The model under review builds one solid part; all positions refer to its coordinate system, in mm. Round coordinates to 2 decimals unless told otherwise and drop trailing zeros. Loops run counter-clockwise (first coordinate to the right, second up) from the corner with the lowest first, then second, coordinate; pieces in that order, holes last. Notation, with made-up numbers: (23.25, 60) - (43.25, 60) arc R25 ccw to (43.25, 95) - close; hole circle Ø6 at (-37.5, 61). An arc over 180 degrees is marked (long way). Answer as CSV lines item,"result".
from build123d import *

# Parameters (mm, degrees)
F0_R     = 76.194135209
F1_DEPTH = 15.24
F2_DEPTH = 15.24
F3_R     = 5.08
F5_DEPTH = 0.762
F6_R     = 71.114135209
F7_DEPTH = 0.254


with BuildPart() as f1:
    # F0 (on Front) → F1 (new body)
    with BuildSketch(Plane.XZ):
        Circle(F0_R)
    extrude(amount=F1_DEPTH)

    # F2 (add): a face of the model
    f2_faces = [f1.faces().sort_by_distance(p)[0] for p in [
        (0, 0, 0),
    ]]
    extrude(f2_faces, amount=F2_DEPTH)

    # F3
    f3_edges = [f1.edges().sort_by_distance(p)[0] for p in [
        (76.194135, -7.62, 0),
        (-76.194135, 0, 0),
        (-76.194135, -15.24, 0),
        (76.194135, 7.62, 0),
        (-76.194135, 15.24, 0),
    ]]
    fillet(f3_edges, radius=F3_R)

    # F4 (on face) → F5 (join)
    with BuildSketch(Plane.XZ.offset(15.24)):
        with BuildLine():
            Line((61.5866476591, -35.5570676045), (0, 0))
            Line((0, 0), (-61.5866476591, -35.5570676045))
            ThreePointArc((-61.5866476591, -35.5570676045), (0, -71.114135209), (61.5866476591, -35.5570676045))
        make_face()
        with BuildLine():
            Line((-61.5866476591, -35.5570676045), (0, 0))
            Line((0, 0), (0, 71.114135209))
            ThreePointArc((0, 71.114135209), (-61.5866476591, 35.5570676045), (-61.5866476591, -35.5570676045))
        make_face()
        with BuildLine():
            Line((0, 71.114135209), (0, 0))
            Line((0, 0), (61.5866476591, -35.5570676045))
            ThreePointArc((61.5866476591, -35.5570676045), (68.6909798125, -18.4056925681), (71.114135209, 0))
            ThreePointArc((71.114135209, 0), (50.2852872445, 50.2852872445), (0, 71.114135209))
        make_face()
    extrude(amount=F5_DEPTH)

    # F6 (on face) → F7 (join)
    with BuildSketch(Plane(origin=(0, 15.24, 0), x_dir=(-1, 0, 0), z_dir=(0, 1, 0))):
        Circle(F6_R)
    extrude(amount=F7_DEPTH)


solid = f1.part
1. Take a section at A-A (y = -4.5). State the section outline as (x, z) points, plus the area to 3 significant figures.
Numbers:
outline,"circle Ø152.39 at (0, 0)"
area,"18,200 mm²"
2. Wall thickness on probe 1 along X at (y, z) = (2.5, -2); probe 2 along Z at (x, y) = (-29.5, 6); probe 3 along Z at (x, y) = (-63, 1): over which ranges is each line inside the solid? List them lowest first.
Numbers:
probe 1,"x = -76.17 to 76.17"
probe 2,"z = -70.25 to 70.25"
probe 3,"z = -42.85 to 42.85"
3. Take a section at B-B (y = 13). State the section outline as (x, z) points, plus the area to 3 significant figures.
Numbers:
outline,"circle Ø150.65 at (0, 0)"
area,"17,800 mm²"
4. Clearance check with flat-ended pins moving along their axes: pin 1 (2 mm diameter, centred on x = -48, y = 4, fed in from +Z); pin 2 (12 mm diameter, centred on y = 10, z = 16, fed in from -X); pin 3 (2 mm diameter, centred on x = 21, y = 9.5, fed in from +Z). State where each tip first meets the part, or that it passes through.
Numbers:
pin 1,"stops at z = 59.97"
pin 2,"stops at x = -75.54"
pin 3,"stops at z = 73.52"
